Geometry: final body of the model. Coordinates: model frame, mm. A direction names the side the tool comes from. Round coordinates to 2 decimals unless told otherwise and drop trailing zeros. Write each loop counter-clockwise with the first axis right and the second up, starting at its lowest first coordinate (ties: lowest second). Pieces come first, ordered by that corner, then holes. Notation, with made-up numbers: M 84,17.25 L 120,17.25 A26 cw 120,56.25 Z; hole C 25,-14 d10. An arc over 180 degrees is marked long. Use one line per item in the form item = value. Start each with the question number.
Item 1: Pin query (flat end, axial travel): pin 1 Ø1.9 at (x, y) = (-9, 10) entering from +Z; pin 2 Ø3 at (x, y) = (17, 9.5) entering from -Z; pin 3 Ø2 at (x, z) = (-33, 38.5) entering from +Y; pin 4 Ø7 at (y, z) = (11, 5.5) entering from -X. Return the tip coordinate at first contact, or that it passes through.
Item 2: Reachability of faces 5 (the cylindrical face through (-71.054, 9.569, -97.781)), 6 (the cylindrical face through (66.416, 13.639, -93.439)), 7 (the flat face through (-1, 9, 101.6)), 8 (the cylindrical face through (-75.594, 14.283, 102.221)), 9 (the flat face through (-1, 9, 99.06)) from +Z, -Z, +X, -X, +Y, -Y: full face, straight path, thin tool, end or side. Return the list, or none.
Item 3: Pull-direction query (Y, two-part tool) for faces 1 (the flat face through (-1, 9, -99.06)), 2 (the flat face through (0, 12.7, -96)), 3 (the cylindrical face through (-71.054, 9.569, 97.781)), 4 (the flat face through (-1, 0, -1)); classes: pulls with the +Y half, pulls with the -Y half, needs draft (parallel to the pull), parting line crosses it, or undercut.
Item 4: Ray query, probe 1 along X at (y, z) = (14, -3); probe 2 along Z at (x, y) = (54.5, 11.5); probe 3 along X at (y, z) = (6.75, -42). Return the intervals inside material, ascending.
Item 5: Section query B-B (z = 53.5). Return loops of the section in (x, y) (3 decimals).
Item 6: Section query A-A (x = -12.5). Return loops of the section in (y, z) (3 decimals).
from build123d import *

# Parameters (mm, degrees)
SKETCH1_W           = 149.352
SKETCH1_H           = 203.2
BOSS_EXTRUDE1_DEPTH = 12.7
FILLET1_R           = 12.7
FILLET3_R           = 6.35
SHELL1_T            = -2.54
BOSS_EXTRUDE2_DEPTH = 3.175
FILLET2_R           = 1.27


with BuildPart() as part:
    # Sketch1 → Boss-Extrude1 (new body)
    with BuildSketch(Plane(origin=(0, 0, 0), x_dir=(1, 0, 0), z_dir=(0, 1, 0))):
        Rectangle(SKETCH1_W, SKETCH1_H)
    extrude(amount=BOSS_EXTRUDE1_DEPTH)

    # Fillet1
    fillet1_edges = [part.edges().sort_by_distance(p)[0] for p in [
        (74.676, 6.35, 101.6),
        (-74.676, 6.35, 101.6),
        (-74.676, 6.35, -101.6),
        (74.676, 6.35, -101.6),
    ]]
    fillet(fillet1_edges, radius=FILLET1_R)

    # Fillet3
    fillet3_edges = [part.edges().sort_by_distance(p)[0] for p in [
        (-74.676, 0, 0),
        (74.676, 0, 0),
        (0, 0, 101.6),
        (0, 0, -101.6),
        (70.956256121, 0, 97.880256121),
        (70.956256121, 0, -97.880256121),
        (-70.956256121, 0, 97.880256121),
        (-70.956256121, 0, -97.880256121),
    ]]
    fillet(fillet3_edges, radius=FILLET3_R)

    # Shell1
    shell1_openings = [part.faces().sort_by_distance(p)[0] for p in [
        (0, 12.7, 0),
    ]]
    offset(amount=SHELL1_T, openings=shell1_openings, kind=Kind.INTERSECTION)

    # Sketch2 → Boss-Extrude2 (add)
    with BuildSketch(Plane(origin=(0, 12.7, 0), x_dir=(1, 0, 0), z_dir=(0, 1, 0))):
        with BuildLine():
            Line((61.976, 107.95), (-61.976, 107.95))
            ThreePointArc((-61.976, 107.95), (-75.446384182, 102.370384182), (-81.026, 88.9))
            Line((-81.026, 88.9), (-81.026, -88.9))
            ThreePointArc((-81.026, -88.9), (-75.446384182, -102.370384182), (-61.976, -107.95))
            Line((-61.976, -107.95), (61.976, -107.95))
            ThreePointArc((61.976, -107.95), (75.446384182, -102.370384182), (81.026, -88.9))
            Line((81.026, -88.9), (81.026, 88.9))
            ThreePointArc((81.026, 88.9), (75.446384182, 102.370384182), (61.976, 107.95))
        make_face()
        with BuildLine():
            Line((-68.326, -88.9), (-68.326, 88.9))
            ThreePointArc((-68.326, 88.9), (-66.466128061, 93.390128061), (-61.976, 95.25))
            Line((-61.976, 95.25), (61.976, 95.25))
            ThreePointArc((61.976, 95.25), (66.466128061, 93.390128061), (68.326, 88.9))
            Line((68.326, 88.9), (68.326, -88.9))
            ThreePointArc((68.326, -88.9), (66.466128061, -93.390128061), (61.976, -95.25))
            Line((61.976, -95.25), (-61.976, -95.25))
            ThreePointArc((-61.976, -95.25), (-66.466128061, -93.390128061), (-68.326, -88.9))
        make_face(mode=Mode.SUBTRACT)
    extrude(amount=BOSS_EXTRUDE2_DEPTH)

    # Fillet2
    fillet2_edges = [part.edges().sort_by_distance(p)[0] for p in [
        (-81.026, 15.875, 0),
        (-75.446384182, 15.875, 102.370384182),
        (0, 15.875, 107.95),
        (75.446384182, 15.875, 102.370384182),
        (81.026, 15.875, 0),
        (75.446384182, 12.7, -102.370384182),
        (0, 12.7, -107.95),
        (-75.446384182, 12.7, -102.370384182),
        (-81.026, 12.7, 0),
        (-75.446384182, 12.7, 102.370384182),
        (0, 12.7, 107.95),
        (75.446384182, 12.7, 102.370384182),
        (81.026, 12.7, 0),
        (-66.466128061, 15.875, 93.390128061),
        (0, 15.875, 95.25),
        (66.466128061, 15.875, 93.390128061),
        (68.326, 15.875, 0),
        (66.466128061, 15.875, -93.390128061),
        (0, 15.875, -95.25),
        (-66.466128061, 15.875, -93.390128061),
        (-68.326, 15.875, 0),
        (75.446384182, 15.875, -102.370384182),
        (0, 15.875, -107.95),
        (-75.446384182, 15.875, -102.370384182),
    ]]
    fillet(fillet2_edges, radius=FILLET2_R)


solid = part.part
Working result:
q1.pin_1 = 101.6
q1.pin_2 = -101.6
q1.pin_3 = 2.54
q1.pin_4 = -81.03
q2.face_5 = -Z, -X, -Y
q2.face_6 = +Y
q2.face_7 = +Z, +X, -X, -Y
q2.face_8 = +Z, -X, +Y, -Y
q2.face_9 = none
q3.face_1 = undercut
q3.face_2 = undercut
q3.face_3 = needs draft
q3.face_4 = pulls with the -Y half
q4.probe_1 = -81.03 to -68.33, 68.33 to 81.03
q4.probe_2 = -101.6 to -99.06, 99.06 to 101.6
q4.probe_3 = -74.68 to -72.14, 72.14 to 74.68
q5.outline = M -81.026,13.97 A1.27 ccw -79.756,12.7 L -74.676,12.7 L -74.676,6.35 A6.35 ccw -68.326,0 L 68.326,0 A6.35 ccw 74.676,6.35 L 74.676,12.7 L 79.756,12.7 A1.27 ccw 81.026,13.97 L 81.026,14.605 A1.27 ccw 79.756,15.875 L 69.596,15.875 A1.27 ccw 68.326,14.605 L 68.326,12.7 L 72.136,12.7 L 72.136,6.35 A3.81 cw 68.326,2.54 L -68.326,2.54 A3.81 cw -72.136,6.35 L -72.136,12.7 L -68.326,12.7 L -68.326,14.605 A1.27 ccw -69.596,15.875 L -79.756,15.875 A1.27 ccw -81.026,14.605 Z
q6.outline = M 0,-95.25 A6.35 ccw 6.35,-101.6 L 12.7,-101.6 L 12.7,-106.68 A1.27 ccw 13.97,-107.95 L 14.605,-107.95 A1.27 ccw 15.875,-106.68 L 15.875,-96.52 A1.27 ccw 14.605,-95.25 L 12.7,-95.25 L 12.7,-99.06 L 6.35,-99.06 A3.81 cw 2.54,-95.25 L 2.54,95.25 A3.81 cw 6.35,99.06 L 12.7,99.06 L 12.7,95.25 L 14.605,95.25 A1.27 ccw 15.875,96.52 L 15.875,106.68 A1.27 ccw 14.605,107.95 L 13.97,107.95 A1.27 ccw 12.7,106.68 L 12.7,101.6 L 6.35,101.6 A6.35 ccw 0,95.25 Z
